Check sheet for the modelled part. Datum: model origin and axes. Units: mm. Coordinates: 2 decimals unless noted, no trailing zeros. Order: outer loops, then holes, each group sorted by start corner. A loop starts at its lowest first (then second) coordinate and runs counter-clockwise, first axis right, second up.
from build123d import *

# Parameters (mm, degrees)
F0_R     = 6.25
F0_R_2   = 3.75
F1_DEPTH = 47
F2_R     = 1


with BuildPart() as f1:
    # F0 (on Right) → F1 (new body)
    with BuildSketch(Plane.YZ):
        Circle(F0_R)
        Circle(F0_R_2, mode=Mode.SUBTRACT)
    extrude(amount=F1_DEPTH)

    # F2
    f2_edges = [f1.edges().sort_by_distance(p)[0] for p in [
        (0, -6.25, 0),
        (0, -3.75, 0),
        (47, -6.25, 0),
        (47, -3.75, 0),
    ]]
    fillet(f2_edges, radius=F2_R)


solid = f1.part
(1) Cross-section at C-C (x = 27). Enter the section's corners in (y, z).
Filled in:
outline: circle Ø12.5 at (0, 0); hole circle Ø7.5 at (0, 0)
(2) Go/stop test with flat-tipped pins: P1, Ø6, axis at x = 35, y = -4.5, coming from the +Z side; P2, Ø5, axis at x = 20, y = -4.5, coming from the +Z side; P3, Ø1, axis at x = 21.5, y = 4, coming from the +Z side. Record where each tip stops, or that it passes through.
Filled in:
P1: stops at z = 6.07
P2: stops at z = 5.92
P3: stops at z = 5.18
(3) Release check for a two-part mould opening along Z. For faces 1 (the flat face through (0, -4, -3)), 2 (the cylindrical face through (23.18, 5.96, 1.88)), 3 (the cylindrical face through (23.185, -3.746, 0.165)) record: +Z half, -Z half, draft (parallel to the pull), parting line (faces both ways), or undercut.
Filled in:
face 1: draft
face 2: parting line
face 3: undercut
(4) Cross-section at A-A (z = 0). Enter the section's corners in (x, y), and give its area (3 significant figures).
Filled in:
outline: (0, -5.25) arc R1 ccw to (1, -6.25) - (46, -6.25) arc R1 ccw to (47, -5.25) - (47, -4.75) arc R1 ccw to (46, -3.75) - (1, -3.75) arc R1 ccw to (0, -4.75) - close; (0, 4.75) arc R1 ccw to (1, 3.75) - (46, 3.75) arc R1 ccw to (47, 4.75) - (47, 5.25) arc R1 ccw to (46, 6.25) - (1, 6.25) arc R1 ccw to (0, 5.25) - close
area: 233 mm2
(5) Thickness scan on probe 1 along Z at (x, y) = (22, 0); probe 2 along Y at (x, z) = (36, -2.5); probe 3 along Z at (x, y) = (11.5, 2.75). Record the ranges inside material, lowest first.
Filled in:
probe 1: z = -6.25 to -3.75, 3.75 to 6.25
probe 2: y = -5.73 to -2.8, 2.8 to 5.73
probe 3: z = -5.61 to -2.55, 2.55 to 5.61
